from build123d import *

# Parameters (mm, degrees)
SKETCH1_R           = 2.5
BOSS_EXTRUDE1_DEPTH = 0.1


with BuildPart() as part:
    # Sketch1 → Boss-Extrude1 (new body)
    with BuildSketch(Plane(origin=(0, 0, 0), x_dir=(1, 0, 0), z_dir=(0, 1, 0))):
        with BuildLine():
            Line((0, 0), (-101.873461229, -2.564384609))
            ThreePointArc((-101.873461229, -2.564384609), (-103.606717283, -5), (-101.873461229, -7.435615391))
            Line((-101.873461229, -7.435615391), (0, -10))
            ThreePointArc((0, -10), (4.075949785, -5), (0, 0))
        make_face()
        with Locations((-1.028794979, -5)):
            Circle(SKETCH1_R, mode=Mode.SUBTRACT)
    extrude(amount=BOSS_EXTRUDE1_DEPTH)


solid = part.part
Input: part model. Units: mm. Frame: model coordinates. Coordinates: 2 decimals unless noted, no trailing zeros. Write each loop counter-clockwise with the first axis right and the second up, starting at its lowest first coordinate (ties: lowest second). Pieces come first, ordered by that corner, then holes. Notation, with made-up numbers: M 37,-15.75 L 91,-15.75 A21 ccw 91,17.25 Z; hole C -8,60.5 d9. An arc over 180 degrees is marked long. Answer as a JSON object with one key per item and string values. Group by question number.
(1) Section B-B on y = 0.05. Output: boundary loops of the cut face in (x, z), plus the area to 3 significant figures.
(2) Ray query, line 1 along X through (y, z) = (0.05, 4); line 2 along Z through (x, y) = (-39.5, 0.05). Return the intervals inside material, ascending. Write a range as [from, to].
(3) Contact query for a flat-ended pin moving along its axis: P1, Ø3, axis at x = -1.03, z = 5, coming from the -Y side. Output: stop coordinate, or through.
(4) Section C-C on x = -40. Output: boundary loops of the cut face in (y, z).
(5) Section D-D on x = -19.5. Output: boundary loops of the cut face in (y, z), plus the area to 3 significant figures.
(6) Section A-A on z = 5. Output: boundary loops of the cut face in (x, y).
Result set:
{
 "1": {"outline": "M -101.87,2.56 L 0,0 A5.1 ccw 0,10 L -101.87,7.44 A2.58 ccw Z; hole C -1.03,5 d5", "area": "775 mm2"},
 "2": {"line 1": "x = [-103.4, -3.32], [1.26, 3.98]", "line 2": "z = [0.99, 9.01]"},
 "3": {"P1": "passes through"},
 "4": {"outline": "M 0,1.01 L 0.1,1.01 L 0.1,8.99 L 0,8.99 Z"},
 "5": {"outline": "M 0,0.49 L 0.1,0.49 L 0.1,9.51 L 0,9.51 Z", "area": "0.902 mm2"},
 "6": {"outline": "M -103.61,0 L -3.53,0 L -3.53,0.1 L -103.61,0.1 Z; M 1.47,0 L 4.08,0 L 4.08,0.1 L 1.47,0.1 Z"}
}
